Autodesk Inventor part; units mm, degrees
ref_plane "P1_XY" through (0, 0, 0) normal (1, 0, 0) x (0, 0, -1)
ref_plane "P1_YZ" through (0, 0, 0) normal (0, 0, -1) x (0, 1, 0)
ref_plane "P1_ZX" through (0, 0, 0) normal (0, 1, 0) x (1, 0, 0)
sketch "Skizze_1" plane through (0, 0, 0) normal (0, 0, 1) x (1, 0, 0)
  line L0 (51, 0) -> (-38, 0)
  line L1 (-38, 0) -> (-38, 2.3865)
  line L2 (-38, 2.3865) -> (-37.3865, 3)
  line L3 (-37.3865, 3) -> (-25.0135, 3)
  line L4 (-25.0135, 3) -> (-24.4, 2.3865)
  line L5 (-24.4, 2.3865) -> (-22, 2.3865)
  line L6 (-22, 2.3865) -> (-22, 3)
  line L7 (-22, 3) -> (48, 3)
  line L8 (48, 3) -> (48, 5.6)
  line L9 (48, 5.6) -> (51, 5.6)
  line L10 (51, 5.6) -> (51, 0)
  line L11 (51, 0) -> (-38, 0)
revolve "Revolution1" add sketch "Skizze_1" angle 360 about axis through (51, 0, 0) along (1, 0, 0)
thread "Thread1"
sketch "Skizze_4" plane through (-22, 0, 0) normal (1, 0, 0) x (0, 0, -1)
  line L0 (-5, -16) -> (5, -16)
  line L1 (5, -16) -> (5, 16)
  line L2 (5, 16) -> (-5, 16)
  line L3 (-5, 16) -> (-5, -16)
  line L4 (-2.5, -8) -> (2.5, -8)
  line L5 (2.5, -8) -> (2.5, 8)
  line L6 (2.5, 8) -> (-2.5, 8)
  line L7 (-2.5, 8) -> (-2.5, -8)
extrude "Extrusion1" cut sketch "Skizze_4" along normal blind 4
ref_plane "P1_XY" through (0, 0, 0) normal (1, 0, 0) x (0, 0, -1)
ref_plane "P1_YZ" through (0, 0, 0) normal (0, 0, -1) x (0, 1, 0)
ref_plane "P1_ZX" through (0, 0, 0) normal (0, 1, 0) x (1, 0, 0)
ref_plane "PD1_XY" through (-32, 0, 0) normal (1, 0, 0) x (0, 0, -1)
ref_plane "PD1_YZ" through (-32, 0, 0) normal (0, 0, -1) x (0, 1, 0)
ref_plane "PD1_ZX" through (-32, 0, 0) normal (0, 1, 0) x (1, 0, 0)
ref_plane "PD2_XY" through (102, 0, 0) normal (1, 0, 0) x (0, 0, -1)
ref_plane "PD2_YZ" through (102, 0, 0) normal (0, 0, -1) x (0, 1, 0)
ref_plane "PD2_ZX" through (102, 0, 0) normal (0, 1, 0) x (1, 0, 0)
properties part number "16N2A12A010-(N0-pistone)"
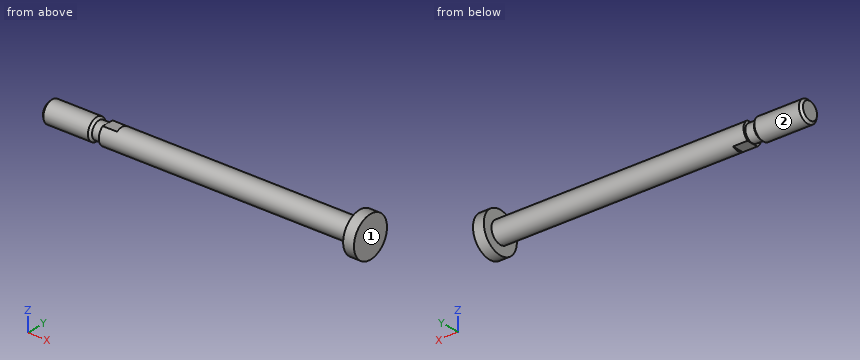
CAD build for the part. Positions are in the model's coordinates, mm. Face numbers are marked on the shaded views. A direction names the side the tool comes from. Give positions to 0.01 mm unless a question says otherwise; leave off trailing zeros. Loops run counter-clockwise (first coordinate to the right, second up) from the corner with the lowest first, then second, coordinate; pieces in that order, holes last. Notation, with made-up numbers: M 80.25,82.25 L 100.25,82.25 A23 cw 100.25,97.25 Z; hole C 11.5,18.5 d4. An arc over 180 degrees is marked long. Use one line per item in the form item = value.
Item 1: Which spindle directions (+Z, -Z, +X, -X, +Y, -Y) get a long thin tool onto all of the face, cutting with end or side? Do the marked faces 1 and 2. Say none if no direction does.
Determined:
face_1 = +Z, -Z, +X, +Y, -Y
face_2 = -X
Item 2: Slice it at B-B (y = 0). List the corners of the cut face in (x, z).
Determined:
outline = M -38,-2.39 L -37.39,-3 L -25.01,-3 L -24.4,-2.39 L -22,-2.39 L -22,-2.5 L -18,-2.5 L -18,-3 L 48,-3 L 48,-5.6 L 51,-5.6 L 51,5.6 L 48,5.6 L 48,3 L -18,3 L -18,2.5 L -22,2.5 L -22,2.39 L -24.4,2.39 L -25.01,3 L -37.39,3 L -38,2.39 Z
Item 3: Slice it at A-A (z = 0). List the corners of the cut face in (x, y), plus the area to 3 significant figures.
Determined:
outline = M -38,-2.39 L -37.39,-3 L -25.01,-3 L -24.4,-2.39 L -22,-2.39 L -22,-3 L 48,-3 L 48,-5.6 L 51,-5.6 L 51,5.6 L 48,5.6 L 48,3 L -22,3 L -22,2.39 L -24.4,2.39 L -25.01,3 L -37.39,3 L -38,2.39 Z
area = 546 mm2
Item 4: Slice it at C-C (x = -31.5). List the corners of the cut face in (y, z).
Determined:
outline = C 0,0 d6
Item 5: Slice it at D-D (y = 4.5). List the corners of the cut face in (x, z).
Determined:
outline = M 48,-3.33 L 51,-3.33 L 51,3.33 L 48,3.33 Z
Item 6: Flat gauge pins, fed straight in: pin 1 (2.5 mm diameter, centred on x = -21, y = 0, fed in from -Z); pin 2 (1 mm diameter, centred on x = -20, y = -0.5, fed in from +Z); pin 3 (1.5 mm diameter, centred on x = 1, z = 1, fed in from -Y). Where does each tip first touch, or does it go through?
Determined:
pin_1 = -2.5
pin_2 = 2.5
pin_3 = -2.99
Item 7: Drill centre lines: probe 1 along X at (y, z) = (-1.5, -3.75); probe 2 along Z at (x, y) = (5.5, -0.25). Where is each one in solid material? Low to high. Write a range as from..to.
Determined:
probe_1 = 48..51
probe_2 = -2.99..2.99
